The drawing under review shows one solid part. Ordinate dimensions are in mm from its lowest x, y, z. A direction names the side the tool comes from. Give positions to 0.01 mm unless a question says otherwise; leave off trailing zeros. Write each loop counter-clockwise with the first axis right and the second up, starting at its lowest first coordinate (ties: lowest second). Pieces come first, ordered by that corner, then holes.
Q1. For line 1 (Y direction, x = 20, z = 1.6); line 2 (Y direction, x = 20, z = 5.75); line 3 (Z direction, x = 34, y = 11), list the stretches that pass through material, from the lowest coordinate up.
Q2. We need section C-C (z = 2.75). Write out the cut boundary in (x, y).
Q3. Mouldability with a two-part tool opening along X and no side actions: class the marked faces 4, 5 and 6 as released by +X, released by -X, zero draft, split by the parting line, or undercut.
Q4. We need section B-B (y = 5). Write out the cut boundary in (x, z), then the cut area to 3 significant figures.
Q5. Machinability: for the marked faces 1, 2 and 3, which of the approach directions +Z, -Z, +X, -X, +Y, -Y give a long, thin tool a straight path to every point of the face, cutting with its end or side? Answer none if there is none.
Q6. We need section A-A (x = 20). Write out the cut boundary in (y, z), then the cut area to 3 significant figures.
Q7. Insertion check: P1, Ø6, axis at x = 26.5, z = 13, coming from the +Y side; P2, Ø6.5, axis at x = 20, y = 20, coming from the -Z side; P3, Ø3, axis at y = 13, z = 2, coming from the +X side; P4, Ø5, axis at x = 11.5, z = 12, coming from the +Y side. Each pin has a flat end and moves straight along its axis. Give the tip position at first contact, or say it passes through.
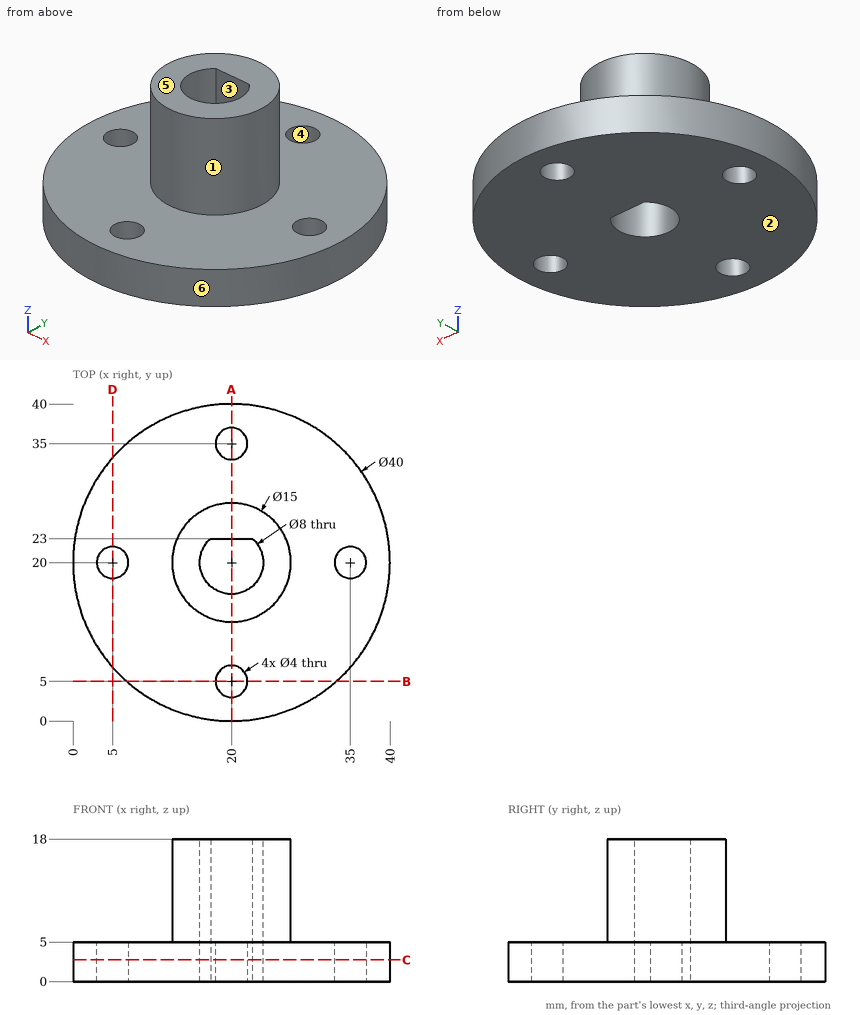
Computed:
1. line 1: y = 0 to 3, 7 to 16, 23 to 33, 37 to 40
1. line 2: y = 12.5 to 16, 23 to 27.5
1. line 3: z = 0 to 5
2. outline: circle Ø40 at (20, 20); hole circle Ø4 at (5, 20); hole (17.35, 23) arc R4 ccw (long way) to (22.65, 23) - close; hole circle Ø4 at (20, 5); hole circle Ø4 at (20, 35); hole circle Ø4 at (35, 20)
3. face 4: undercut
3. face 5: zero draft
3. face 6: split by the parting line
4. outline: (6.77, 0) - (18, 0) - (18, 5) - (6.77, 5) - close; (22, 0) - (33.23, 0) - (33.23, 5) - (22, 5) - close
4. area: 112 mm2
5. face 1: +Z
5. face 2: -Z, +X, -X, +Y, -Y
5. face 3: +Z, -Z
6. outline: (0, 0) - (3, 0) - (3, 5) - (0, 5) - close; (7, 0) - (16, 0) - (16, 18) - (12.5, 18) - (12.5, 5) - (7, 5) - close; (23, 0) - (33, 0) - (33, 5) - (27.5, 5) - (27.5, 18) - (23, 18) - close; (37, 0) - (40, 0) - (40, 5) - (37, 5) - close
6. area: 229 mm2
7. P1: stops at y = 26.63
7. P2: stops at z = 0
7. P3: stops at x = 39.23
7. P4: stops at y = 24.5
